from build123d import *

# Parameters (mm, degrees)
SKETCH_1_W          = 47
SKETCH_1_H          = 30
EXTRUDE_1_DEPTH     = 11
SKETCH_2_R          = 6
EXTRUDE_2_DEPTH     = 3
EXTRUDE_3_DEPTH     = 8
SKETCH_4_R          = 14
EXTRUDE_4_DEPTH     = 50
SKETCH_5_R          = 5
EXTRUDE_5_DEPTH     = 2
SKETCH_6_R          = 1.5
CUT_EXTRUDE_1_DEPTH = 31
CUT_EXTRUDE_2_DEPTH = 48
SKETCH_9_R          = 1.5
CUT_EXTRUDE_3_DEPTH = 8
SKETCH_11_R         = 0.5
EXTRUDE_6_DEPTH     = 8


with BuildPart() as part:
    # 草图1 → 凸台-拉伸1 (new body)
    with BuildSketch(Plane(origin=(0, 0, 0), x_dir=(1, 0, 0), z_dir=(0, 1, 0))):
        with Locations((23.5, -15)):
            Rectangle(SKETCH_1_W, SKETCH_1_H)
    extrude(amount=EXTRUDE_1_DEPTH)

    # 草图2 → 凸台-拉伸2 (add)
    with BuildSketch(Plane(origin=(0, 11, 0), x_dir=(1, 0, 0), z_dir=(0, 1, 0))):
        with Locations((33.5, -15)):
            Circle(SKETCH_2_R)
    extrude(amount=EXTRUDE_2_DEPTH)

    # 草图3 → 凸台-拉伸3 (add)
    with BuildSketch(Plane(origin=(0, 14, 0), x_dir=(1, 0, 0), z_dir=(0, 1, 0))):
        Polygon((37.25277675, -15), (35.376388375, -11.75), (31.623611625, -11.75), (29.74722325, -15), (31.623611625, -18.25), (35.376388375, -18.25), align=None)
    extrude(amount=EXTRUDE_3_DEPTH)

    # 草图4 → 凸台-拉伸4 (add)
    with BuildSketch(Plane.XZ):
        with Locations((16, 15)):
            Circle(SKETCH_4_R)
    extrude(amount=EXTRUDE_4_DEPTH)

    # 草图5 → 凸台-拉伸5 (add)
    with BuildSketch(Plane.XZ.offset(50)):
        with Locations((16, 15)):
            Circle(SKETCH_5_R)
    extrude(amount=EXTRUDE_5_DEPTH)

    # 草图6 → 切除-拉伸1 (cut, through all)
    with BuildSketch(Plane.XY.offset(30)):
        with Locations((3.340757383, 8.25)):
            Circle(SKETCH_6_R)
        with Locations((32.340757383, 8.25)):
            Circle(SKETCH_6_R)
        with Locations((42.840757383, 8.25)):
            Circle(SKETCH_6_R)
    extrude(amount=-CUT_EXTRUDE_1_DEPTH, mode=Mode.SUBTRACT)

    # 草图7 → 切除-拉伸2 (cut, through all)
    with BuildSketch(Plane.ZY):
        with BuildLine():
            Line((11, -37.25), (19, -37.25))
            ThreePointArc((19, -37.25), (20.75, -39), (19, -40.75))
            Line((19, -40.75), (11, -40.75))
            ThreePointArc((11, -40.75), (9.25, -39), (11, -37.25))
        make_face()
    extrude(amount=-CUT_EXTRUDE_2_DEPTH, mode=Mode.SUBTRACT)

    # 草图9 → 切除-拉伸3 (cut)
    with BuildSketch(Plane(origin=(0, 22, 0), x_dir=(1, 0, 0), z_dir=(0, 1, 0))):
        with Locations((33.5, -15)):
            Circle(SKETCH_9_R)
    extrude(amount=-CUT_EXTRUDE_3_DEPTH, mode=Mode.SUBTRACT)

    # 草图11 → 凸台-拉伸6 (add)
    with BuildSketch(Plane.XZ.offset(52)):
        with Locations((16, 15)):
            Circle(SKETCH_11_R)
    extrude(amount=EXTRUDE_6_DEPTH)


solid = part.part
CAD build for the part. Positions are in the model's coordinates, mm. A direction names the side the tool comes from. Round coordinates to 2 decimals unless told otherwise and drop trailing zeros. Write each loop counter-clockwise with the first axis right and the second up, starting at its lowest first coordinate (ties: lowest second). Pieces come first, ordered by that corner, then holes. Notation, with made-up numbers: M 78.25,84.25 L 119.25,84.25 A8 ccw 119.25,96.25 Z; hole C 12,54.25 d3. An arc over 180 degrees is marked long. Put each result on its own line as item: value. Start each with the question number.
1) Drill centre lines: probe 1 along Y at (x, z) = (22.5, 16.75); probe 2 along X at (y, z) = (16, 15); probe 3 along Y at (x, z) = (19.5, 12.5). Where is each one in solid material? Low to high. Write a range as [from, to].
2) Pin check, flat tips, straight feed: pin 1 Ø4 at (x, z) = (15, 14.5) entering from +Y; pin 2 Ø5 at (x, z) = (37, 16.5) entering from -Y; pin 3 Ø2 at (x, y) = (18.5, -24) entering from +Z; pin 4 Ø2.5 at (x, y) = (42.84, 8.25) entering from +Z. Stop position of each tip, or through.
3) Saw through at A-A, the plane y = 15.5. Write the cut outline in (x, z).
4) Saw through at C-C, the plane z = 23. Write the cut outline in (x, y), and give its area (3 significant figures).
5) Pull direction Y, two halves, no side cores. Call faces 1 (the cylindrical face through (18.307, -50.986, 10.564)), 2 (the flat face through (23, 11, 15)), 3 (the cylindrical face through (30.842, 8.316, 15.21)): pulls with the +Y half, pulls with the -Y half, needs draft (parallel to the pull), parting line crosses it, or undercut.
6) Saw through at B-B, the plane x = 7. Write the cut outline in (y, z), and give its area (3 significant figures).
7) 3-axis set-ups, long thin cutter, end or side, ignore diameter. For faces 4 (the cylindrical face through (32.3, 18.1, 15.9)), 5 (the flat face through (33, 18, 18.25)), 6 (the cylindrical face through (15.81, -39.04, 9.25)): which of +Z, -Z, +X, -X, +Y, -Y reach the whole face in a straight line?
8) Saw through at D-D, the plane y = -24.5. Write the cut outline in (x, z).
Resolved:
1. probe 1: [-50, -40.75], [-37.25, 11]
1. probe 2: [29.75, 32], [35, 37.25]
1. probe 3: [-52, -40.75], [-37.25, 11]
2. pin 1: y = 11
2. pin 2: y = 0
2. pin 3: z = 28.92
2. pin 4: through
3. outline: M 29.75,15 L 31.62,11.75 L 35.38,11.75 L 37.25,15 L 35.38,18.25 L 31.62,18.25 Z; hole C 33.5,15 d3
4. outline: M 0,0 L 4.51,0 L 4.51,-50 L 27.49,-50 L 27.49,0 L 47,0 L 47,11 L 0,11 Z; hole C 3.34,8.25 d3; hole C 32.34,8.25 d3; hole C 42.84,8.25 d3
4. area: 1,640 mm²
5. face 1: needs draft
5. face 2: pulls with the +Y half
5. face 3: undercut
6. outline: M -50,4.28 L 0,4.28 L 0,0 L 11,0 L 11,30 L 0,30 L 0,25.72 L -50,25.72 Z; hole M -40.75,11 A1.75 ccw -37.25,11 L -37.25,19 A1.75 ccw -40.75,19 Z
6. area: 1,360 mm²
7. face 4: +Y
7. face 5: +Z, +X, -X, +Y
7. face 6: +X, -X
8. outline: C 16,15 d28
